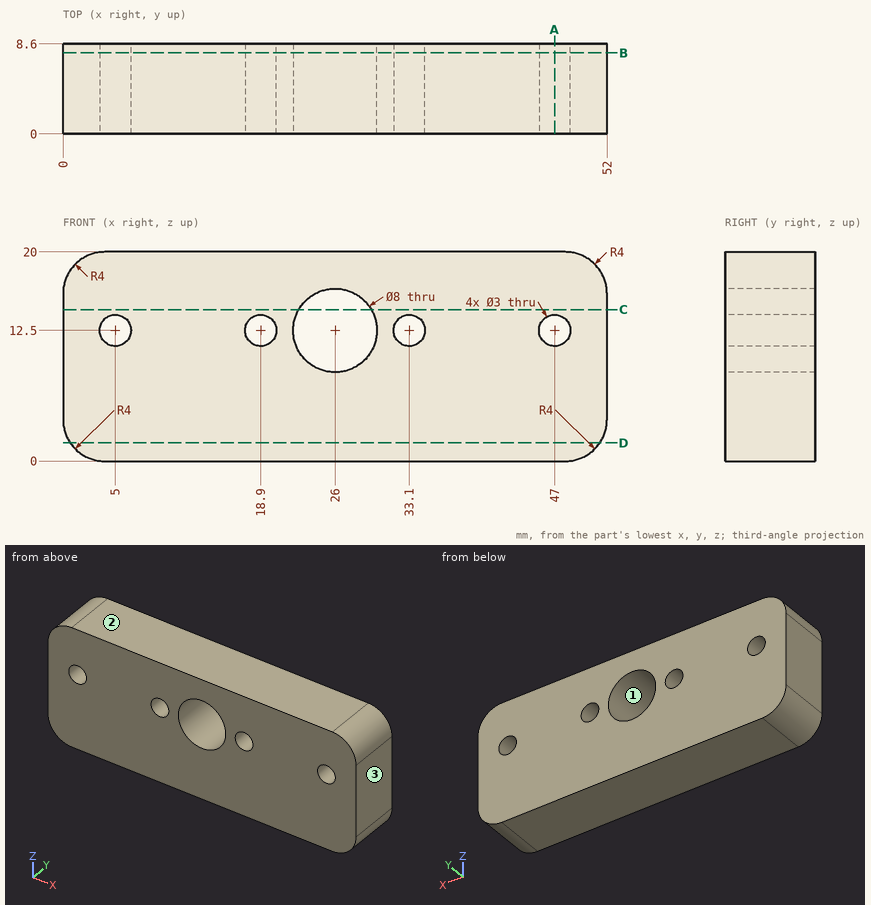
Drawing for the job (mm, zero at the part's lowest x, y, z). Give positions to 0.01 mm unless a question says otherwise; leave off trailing zeros. Loops run counter-clockwise (first coordinate to the right, second up) from the corner with the lowest first, then second, coordinate; pieces in that order, holes last.
1) Band-saw the part on A-A on x = 47. List the corners of the cut face in (y, z).
Values follow:
outline: (0, 0) - (8.6, 0) - (8.6, 11) - (0, 11) - close; (0, 14) - (8.6, 14) - (8.6, 20) - (0, 20) - close
2) Probe line 1 along X through (y, z) = (5.5, 12.5); line 2 along Z through (x, y) = (18.9, 2.25); line 3 along X through (y, z) = (6.5, 15.25). List the from-to ranges inside material, lowest first.
Values follow:
line 1: x = 0 to 3.5, 6.5 to 17.4, 20.4 to 22, 30 to 31.6, 34.6 to 45.5, 48.5 to 52
line 2: z = 0 to 11, 14 to 20
line 3: x = 0 to 23.1, 28.9 to 52
3) Two-plate mould, pull along X, no slides. Class the marked faces 1, 2 and 3: released by +X, released by -X, zero draft, split by the parting line, or undercut.
Values follow:
face 1: undercut
face 2: zero draft
face 3: released by +X
4) Band-saw the part on D-D on z = 1.75. List the corners of the cut face in (x, y), then the cut area to 3 significant figures.
Values follow:
outline: (0.69, 0) - (51.31, 0) - (51.31, 8.6) - (0.69, 8.6) - close
area: 435 mm2
5) Band-saw the part on B-B on y = 7.75. List the corners of the cut face in (x, z).
Values follow:
outline: (0, 4) arc R4 ccw to (4, 0) - (48, 0) arc R4 ccw to (52, 4) - (52, 16) arc R4 ccw to (48, 20) - (4, 20) arc R4 ccw to (0, 16) - close; hole circle Ø3 at (5, 12.5); hole circle Ø3 at (18.9, 12.5); hole circle Ø8 at (26, 12.5); hole circle Ø3 at (33.1, 12.5); hole circle Ø3 at (47, 12.5)
6) Drop flat-ended pins along their axis: P1, Ø2, axis at y = 7, z = 2.5, coming from the +X side; P2, Ø5, axis at x = 47, z = 12.5, coming from the +Y side. Give the stop position or say it passes through.
Values follow:
P1: stops at x = 51.97
P2: stops at y = 8.6
7) Band-saw the part on C-C on z = 14.5. List the corners of the cut face in (x, y), then the cut area to 3 significant figures.
Values follow:
outline: (0, 0) - (22.54, 0) - (22.54, 8.6) - (0, 8.6) - close; (29.46, 0) - (52, 0) - (52, 8.6) - (29.46, 8.6) - close
area: 388 mm2
